The model under review builds one solid part; all positions refer to its coordinate system, in mm. Coordinates: 2 decimals unless noted, no trailing zeros. Order: outer loops, then holes, each group sorted by start corner. A loop starts at its lowest first (then second) coordinate and runs counter-clockwise, first axis right, second up. Notation, with made-up numbers: M 69.5,78.25 L 78.5,78.25 A29 ccw 78.5,101.25 Z; hole C -5.5,63.25 d11. An arc over 180 degrees is marked long. Answer in a Markdown table with one row per item.
from build123d import *

# Parameters (mm, degrees)
BOSS_EXTRUDE1_DEPTH = 3


with BuildPart() as part:
    # Sketch1 → Boss-Extrude1 (new body)
    with BuildSketch(Plane(origin=(0, 0, 0), x_dir=(1, 0, 0), z_dir=(0, 1, 0))):
        Polygon((12, 65.5), (0, 65.5), (0, 59.5), (-3, 59.5), (-3, 39.5), (0, 39.5), (0, 24.5), (-3, 24.5), (-3, 4.5), (0, 4.5), (0, 0), (12, 0), (12, -3), (32, -3), (32, 0), (47, 0), (47, -3), (67, -3), (67, 0), (82, 0), (82, -3), (89, -3), (89, 0), (89, 4.5), (92, 4.5), (92, 24.5), (89, 24.5), (89, 39.5), (92, 39.5), (92, 59.5), (89, 59.5), (89, 65.5), (89, 68.5), (82, 68.5), (82, 65.5), (67, 65.5), (67, 68.5), (47, 68.5), (47, 65.5), (32, 65.5), (32, 68.5), (12, 68.5), align=None)
    extrude(amount=BOSS_EXTRUDE1_DEPTH)


solid = part.part
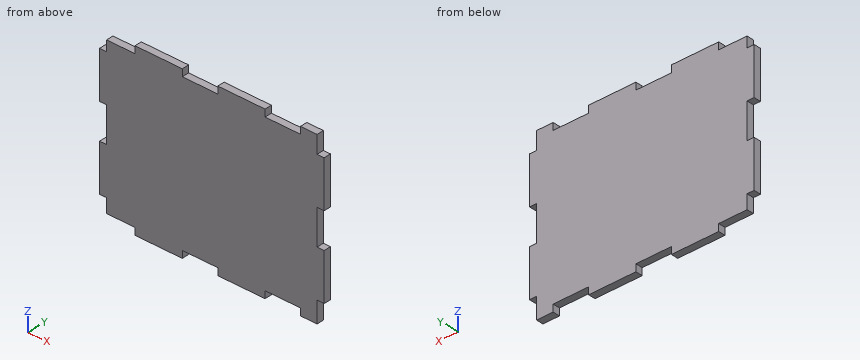
(1) Take a section at B-B (x = 70). Write out the cut boundary in (y, z).
Report:
| item | result |
|---|---|
| outline | M 0,-65.5 L 3,-65.5 L 3,0 L 0,0 Z |
(2) To check wall thickness, follow line 1 (Z direction, x = 10.5, y = 2.65); line 2 (X direction, y = 2.35, z = -29). State the ranges of each line that lie inside material, in increasing order. Write a range as [from, to].
Report:
| item | result |
|---|---|
| line 1 | [-65.5, 0] |
| line 2 | [0, 89] |
(3) Take a section at A-A (z = -1.5). Write out the cut boundary in (x, y), then the cut area to 3 significant figures.
Report:
| item | result |
|---|---|
| outline | M 0,0 L 89,0 L 89,3 L 0,3 Z |
| area | 267 mm^2 |
(4) Insertion check: P1, Ø0.9, axis at y = 2, z = -61.5, coming from the -X side; P2, Ø0.9, axis at y = 1, z = 2, coming from the -X side; P3, Ø1.5, axis at y = 2, z = -67, coming from the +X side. Each pin has a flat end and moves straight along its axis. Give the tip position at first contact, or say it passes through.
Report:
| item | result |
|---|---|
| P1 | x = 0 |
| P2 | x = 12 |
| P3 | x = 89 |
